```python
from build123d import *

# Parameters (mm, degrees)
SKETCH_1_W          = 46.6
SKETCH_1_H          = 43.6
EXTRUDE_1_DEPTH     = 7.4
SKETCH_2_W          = 45
SKETCH_2_H          = 42
CUT_EXTRUDE_1_DEPTH = 6.6
CUT_EXTRUDE_3_REACH = 45.6
SKETCH_3_W          = 20
SKETCH_3_H          = 6.6
FILLET_1_R          = 2


with BuildPart() as part:
    # ｽｹｯﾁ1 → ﾎﾞｽ - 押し出し1 (new body)
    with BuildSketch(Plane.XY):
        Rectangle(SKETCH_1_W, SKETCH_1_H)
    extrude(amount=EXTRUDE_1_DEPTH)

    # ｽｹｯﾁ2 → ｶｯﾄ - 押し出し1 (cut)
    with BuildSketch(Plane.XY.offset(7.4)):
        Rectangle(SKETCH_2_W, SKETCH_2_H)
    extrude(amount=-CUT_EXTRUDE_1_DEPTH, mode=Mode.SUBTRACT)

    # ｽｹｯﾁ3 → ｶｯﾄ - 押し出し3 (cut, up to next)
    with BuildSketch(Plane(origin=(0, -21.8, 0), x_dir=(-1, 0, 0), z_dir=(0, -1, 0)), mode=Mode.PRIVATE) as cut_extrude_3_sk1:
        with Locations((0, -4.1)):
            Rectangle(SKETCH_3_W, SKETCH_3_H)
    cut_extrude_3_tool1 = extrude(cut_extrude_3_sk1.sketch, amount=-CUT_EXTRUDE_3_REACH, mode=Mode.PRIVATE) & part.part
    add(cut_extrude_3_tool1.solids().sort_by_distance((0, -21.8, 4.1))[0], mode=Mode.SUBTRACT)

    # ﾌｨﾚｯﾄ1
    fillet_1_edges = [part.edges().sort_by_distance(p)[0] for p in [
        (-22.5, -21, 4.1),
        (-22.5, 21, 4.1),
        (22.5, 21, 4.1),
        (22.5, -21, 4.1),
        (23.3, -21.8, 3.7),
        (-23.3, -21.8, 3.7),
        (-23.3, 21.8, 3.7),
        (23.3, 21.8, 3.7),
    ]]
    fillet(fillet_1_edges, radius=FILLET_1_R)


solid = part.part
```
Geometry check sheet. Reference: the model listing, model coordinates, mm. A direction names the side the tool comes from. Give positions to 0.01 mm unless a question says otherwise; leave off trailing zeros. Order: outer loops, then holes, each group sorted by start corner. A loop starts at its lowest first (then second) coordinate and runs counter-clockwise, first axis right, second up.
1. Thickness scan on L1, parallel to X at y = 8, z = 2.75; L2, parallel to Y at x = -14, z = 4.75; L3, parallel to Y at x = -7.5, z = 4.5. Record the ranges inside material, lowest first.
2. Release check for a two-part mould opening along Y. For faces 1 (the face through (0, 21, 4)), 2 (the face through (0, 0, 0)), 3 (the face through (-22.73, -21.2, 3.75)) record: pulls with the +Y half, pulls with the -Y half, needs draft (parallel to the pull), parting line crosses it, or undercut.
3. Gauge pin test, flat ends, axial feed: pin 1 Ø8 at (x, y) = (1, 17.5) entering from +Z; pin 2 Ø2 at (x, z) = (-8.5, 2.5) entering from -Y; pin 3 Ø5 at (x, y) = (7.5, -9.5) entering from +Z. Record the tip position at first contact, or that the pin passes through.
4. Section check C-C, the plane x = 12.5. Enter the section's corners in (y, z).
5. Section check B-B, the plane y = -15. Enter the section's corners in (x, z).
6. Section check A-A, the plane z = 3.75. Enter the section's corners in (x, y).
7. Access from +Z, -Z, +X, -X, +Y, -Y to the whole of each face (thin tool, end or side, straight path). Record for faces 4 (the face through (-22.73, 21.2, 3.75)), 5 (the face through (15, -21, 4)).
8. Section check D-D, the plane x = 6.5. Enter the section's corners in (y, z), and give its area (3 significant figures).
Values follow:
1. L1: x = -23.3 to -22.5, 22.5 to 23.3
1. L2: y = -21.8 to -21, 21 to 21.8
1. L3: y = 21 to 21.8
2. face 1: undercut
2. face 2: needs draft
2. face 3: pulls with the -Y half
3. pin 1: stops at z = 7.4
3. pin 2: stops at y = 21
3. pin 3: stops at z = 0.8
4. outline: (-21.8, 0) - (21.8, 0) - (21.8, 7.4) - (21, 7.4) - (21, 0.8) - (-21, 0.8) - (-21, 7.4) - (-21.8, 7.4) - close
5. outline: (-23.3, 0) - (23.3, 0) - (23.3, 7.4) - (22.5, 7.4) - (22.5, 0.8) - (-22.5, 0.8) - (-22.5, 7.4) - (-23.3, 7.4) - close
6. outline: (-23.3, -19.8) arc R2 ccw to (-21.3, -21.8) - (-10, -21.8) - (-10, -21) - (-20.5, -21) arc R2 cw to (-22.5, -19) - (-22.5, 19) arc R2 cw to (-20.5, 21) - (20.5, 21) arc R2 cw to (22.5, 19) - (22.5, -19) arc R2 cw to (20.5, -21) - (10, -21) - (10, -21.8) - (21.3, -21.8) arc R2 ccw to (23.3, -19.8) - (23.3, 19.8) arc R2 ccw to (21.3, 21.8) - (-21.3, 21.8) arc R2 ccw to (-23.3, 19.8) - close
7. face 4: +Z, -Z, -X, +Y
7. face 5: +Z
8. outline: (-21.8, 0) - (21.8, 0) - (21.8, 7.4) - (21, 7.4) - (21, 0.8) - (-21.8, 0.8) - close
8. area: 40.2 mm2
